Here's how the part is built. I have some questions about the finished solid (model axes, mm). A direction names the side the tool comes from. Give positions to 0.01 mm unless a question says otherwise; leave off trailing zeros. Loops run counter-clockwise (first coordinate to the right, second up) from the corner with the lowest first, then second, coordinate; pieces in that order, holes last. Notation, with made-up numbers: (88.25, -21.5) - (134.25, -21.5) arc R14 ccw to (134.25, 1.5) - close; hole circle Ø2 at (-20, 48). An arc over 180 degrees is marked (long way). Use one line per item in the form item = value.
from build123d import *

# Parameters (mm, degrees)
CROQUIS1_R              = 3
SALIENTE_EXTRUIR1_DEPTH = 3
CORTAR_EXTRUIR1_DEPTH   = 3


with BuildPart() as part:
    # Croquis1 → Saliente-Extruir1 (new body)
    with BuildSketch(Plane.XY):
        Polygon((-15, -28.345), (15, -28.345), (15, 28.345), (10, 28.345), (10, 25.345), (5, 25.345), (5, 28.345), (0, 28.345), (0, 25.345), (-5, 25.345), (-5, 28.345), (-10, 28.345), (-10, 25.345), (-15, 25.345), align=None)
        with Locations((0, -18.345)):
            Circle(CROQUIS1_R, mode=Mode.SUBTRACT)
    extrude(amount=SALIENTE_EXTRUIR1_DEPTH)

    # Croquis2 → Cortar-Extruir1 (cut)
    with BuildSketch(Plane(origin=(0, 0, 0), x_dir=(-1, 0, 0), z_dir=(0, 0, -1))):
        with BuildLine():
            Line((-15, -18.345), (-21.186751232, -18.345))
            Line((-21.186751232, -18.345), (-21.186751232, -37.148085908))
            Line((-21.186751232, -37.148085908), (21.188955731, -37.148085908))
            Line((21.188955731, -37.148085908), (21.188955731, -18.345))
            Line((21.188955731, -18.345), (15, -18.345))
            ThreePointArc((15, -18.345), (0, -33.345), (-15, -18.345))
        make_face()
    extrude(amount=-CORTAR_EXTRUIR1_DEPTH, mode=Mode.SUBTRACT)


solid = part.part
(1) If we section it at C-C (y = -22): List the corners of the cut face in (x, z) for me, plus the area to 3 significant figures.
Geometry says:
outline = (-14.55, 0) - (14.55, 0) - (14.55, 3) - (-14.55, 3) - close
area = 87.3 mm²
(2) Thinking about a two-plate mould opening in X: for faces 4 (the flat face through (-10, 27, 1)), 5 (the flat face through (15, 5, 1)), 6 (the cylindrical face through (-0.65, -21.274, 1.479)), which applies, pulls with the +X half, pulls with the -X half, needs draft (parallel to the pull), parting line crosses it, or undercut?
Geometry says:
face_4 = pulls with the -X half
face_5 = pulls with the +X half
face_6 = undercut
(3) If we section it at B-B (x = 7): List the corners of the cut face in (y, z) for me (3 decimals).
Geometry says:
outline = (-28.345, 0) - (25.345, 0) - (25.345, 3) - (-28.345, 3) - close
(4) If we section it at A-A (z = 0.7): List the corners of the cut face in (x, y) for me (3 decimals), plus the area to 3 significant figures.
Geometry says:
outline = (-15, -18.345) arc R15 ccw to (-11.18, -28.345) - (11.18, -28.345) arc R15 ccw to (15, -18.345) - (15, 28.345) - (10, 28.345) - (10, 25.345) - (5, 25.345) - (5, 28.345) - (0, 28.345) - (0, 25.345) - (-5, 25.345) - (-5, 28.345) - (-10, 28.345) - (-10, 25.345) - (-15, 25.345) - close; hole circle Ø6 at (0, -18.345)
area = 1,600 mm²
(5) If I drill on probe 1 along X at (y, z) = (-18.5, 2.3); probe 2 along X at (y, z) = (26.5, 0.4); probe 3 along Y at (x, z) = (9, 0.75) (3 decimals), over which ranges is the centre line in solid material (lowest first)?
Geometry says:
probe_1 = -15 to -3, 3 to 15
probe_2 = -10 to -5, 0 to 5, 10 to 15
probe_3 = -28.345 to 25.345
(6) For P1, Ø1.5, axis at x = 8.5, z = 1.5, coming from the +Y side (3 decimals); P2, Ø1.5, axis at y = 27, z = 2, coming from the -X side, each with a flat end and sliding along its axis, tell me the tip position at first contact or that it passes through.
Geometry says:
P1 = 25.345
P2 = -10
(7) For faces 1 (the flat face through (-2, 25.345, 1)), 2 (the flat face through (0, -28.345, 1)), 3 (the flat face through (-12, 25.345, 1)), which set-ups out of +Z, -Z, +X, -X, +Y, -Y let a thin tool reach every point of the face, with its end or its side?
Geometry says:
face_1 = +Z, -Z, +Y
face_2 = +Z, -Z, +X, -X, -Y
face_3 = +Z, -Z, -X, +Y
